Build history of the part. All positions in model axes, mm. Round coordinates to 2 decimals unless told otherwise and drop trailing zeros. Write each loop counter-clockwise with the first axis right and the second up, starting at its lowest first coordinate (ties: lowest second). Pieces come first, ordered by that corner, then holes. Notation, with made-up numbers: (24, 23.5) -> (46, 23.5) arc R18 ccw to (46, 33.5) -> close; hole circle Ø8 at (29, 74.5). An arc over 180 degrees is marked (long way). Return JSON: item names as keys, results as strings.
from build123d import *

# Parameters (mm, degrees)
SKETCH1_R           = 3.9
SKETCH1_R_2         = 3
SKETCH1_R_3         = 1.95
SKETCH1_R_4         = 3.5
SKETCH1_R_5         = 1.475
BOSS_EXTRUDE2_DEPTH = 5


with BuildPart() as part:
    # Sketch1 → Boss-Extrude2 (new body)
    with BuildSketch(Plane.XY):
        with BuildLine():
            Line((-40, -65), (95, -65))
            ThreePointArc((95, -65), (102.071067812, -62.071067812), (105, -55))
            Line((105, -55), (105, 55))
            ThreePointArc((105, 55), (102.071067812, 62.071067812), (95, 65))
            Line((95, 65), (-40, 65))
            ThreePointArc((-40, 65), (-105, 0), (-40, -65))
        make_face()
        with Locations((95, 55)):
            Circle(SKETCH1_R, mode=Mode.SUBTRACT)
        with Locations((95, -55)):
            Circle(SKETCH1_R, mode=Mode.SUBTRACT)
        with Locations((-90, 0)):
            Circle(SKETCH1_R, mode=Mode.SUBTRACT)
        with Locations((-40, -18)):
            Circle(SKETCH1_R_2, mode=Mode.SUBTRACT)
        with Locations((-40, 18)):
            Circle(SKETCH1_R_2, mode=Mode.SUBTRACT)
        with Locations((80, 40)):
            Circle(SKETCH1_R_3, mode=Mode.SUBTRACT)
        with Locations((80, -40)):
            Circle(SKETCH1_R_3, mode=Mode.SUBTRACT)
        with Locations((-70, 40)):
            Circle(SKETCH1_R_3, mode=Mode.SUBTRACT)
        with Locations((-70, -40)):
            Circle(SKETCH1_R_3, mode=Mode.SUBTRACT)
        with Locations((47, 42.5)):
            Circle(SKETCH1_R_4, mode=Mode.SUBTRACT)
        with Locations((97, 42.5)):
            Circle(SKETCH1_R_4, mode=Mode.SUBTRACT)
        with Locations((97, -42.5)):
            Circle(SKETCH1_R_4, mode=Mode.SUBTRACT)
        with Locations((47, -42.5)):
            Circle(SKETCH1_R_4, mode=Mode.SUBTRACT)
        with Locations((-40, 58.5)):
            Circle(SKETCH1_R_5, mode=Mode.SUBTRACT)
        with Locations((-40, -58.5)):
            Circle(SKETCH1_R_5, mode=Mode.SUBTRACT)
        with BuildLine():
            Line((-3.5, 5), (47.5, 5))
            ThreePointArc((47.5, 5), (52.5, 0), (47.5, -5))
            Line((47.5, -5), (-3.5, -5))
            ThreePointArc((-3.5, -5), (-8.5, 0), (-3.5, 5))
        make_face(mode=Mode.SUBTRACT)
        with BuildLine():
            Line((9.5, 23), (34.5, 23))
            ThreePointArc((34.5, 23), (39.5, 18), (34.5, 13))
            Line((34.5, 13), (9.5, 13))
            ThreePointArc((9.5, 13), (4.5, 18), (9.5, 23))
        make_face(mode=Mode.SUBTRACT)
        with BuildLine():
            Line((9.5, -23), (34.5, -23))
            ThreePointArc((34.5, -23), (39.5, -18), (34.5, -13))
            Line((34.5, -13), (9.5, -13))
            ThreePointArc((9.5, -13), (4.5, -18), (9.5, -23))
        make_face(mode=Mode.SUBTRACT)
    extrude(amount=BOSS_EXTRUDE2_DEPTH)


solid = part.part
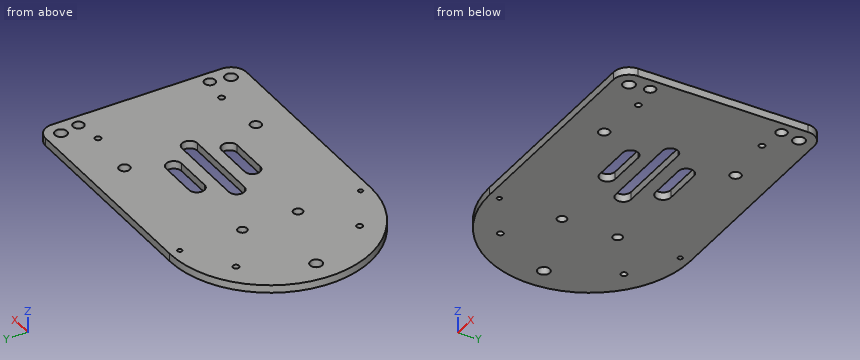
Q1. Wall check: L1, parallel to Y at x = 47, z = 3.3; L2, parallel to Y at x = -40, z = 3.45 (3 decimals); L3, parallel to Y at x = 17, z = 2. Give the ranges that are in metal, low to high.
Verdict:
{"L1": "y = -65 to -46, -39 to -5, 5 to 39, 46 to 65", "L2": "y = -65 to -59.975, -57.025 to -21, -15 to 15, 21 to 57.025, 59.975 to 65", "L3": "y = -65 to -23, -13 to -5, 5 to 13, 23 to 65"}
Q2. Pin check, flat tips, straight feed: pin 1 Ø4.5 at (x, y) = (95, 55) entering from -Z; pin 2 Ø1 at (y, z) = (-44, 4) entering from -X; pin 3 Ø1.5 at (y, z) = (29, 3) entering from -X; pin 4 Ø3 at (y, z) = (-27, 3.5) entering from -X. Stop position of each tip, or through.
Verdict:
{"pin 1": "passes through", "pin 2": "stops at x = -88.3", "pin 3": "stops at x = -98.54", "pin 4": "stops at x = -99.79"}
Q3. Saw through at C-C on y = -18. List the corners of the cut face in (x, z).
Verdict:
{"outline": "(-102.46, 0) -> (-43, 0) -> (-43, 5) -> (-102.46, 5) -> close; (-37, 0) -> (4.5, 0) -> (4.5, 5) -> (-37, 5) -> close; (39.5, 0) -> (105, 0) -> (105, 5) -> (39.5, 5) -> close"}
Q4. Saw through at D-D on x = -90. List the corners of the cut face in (y, z), then the cut area to 3 significant figures.
Verdict:
{"outline": "(-41.53, 0) -> (-3.9, 0) -> (-3.9, 5) -> (-41.53, 5) -> close; (3.9, 0) -> (41.53, 0) -> (41.53, 5) -> (3.9, 5) -> close", "area": "376 mm²"}
Q5. Saw through at A-A on x = 20.5. List the corners of the cut face in (y, z), then the cut area to 3 significant figures.
Verdict:
{"outline": "(-65, 0) -> (-23, 0) -> (-23, 5) -> (-65, 5) -> close; (-13, 0) -> (-5, 0) -> (-5, 5) -> (-13, 5) -> close; (5, 0) -> (13, 0) -> (13, 5) -> (5, 5) -> close; (23, 0) -> (65, 0) -> (65, 5) -> (23, 5) -> close", "area": "500 mm²"}
Q6. Saw through at B-B on z = 1.6. Count the separate pieces of the cut face and the enclosed holes in it, then the cut area to 3 significant figures.
Verdict:
{"separate pieces": "1", "enclosed holes": "18", "area": "23,800 mm²"}
